```python
from build123d import *

# Parameters (mm, degrees)
ESBO_O2_R                = 2.5
ESBO_O2_R_2              = 2
RESSALTO_EXTRUS_O1_DEPTH = 3
ESBO_O3_W                = 5.4
ESBO_O3_H                = 7.4
ESBO_O3_W_2              = 3.4
ESBO_O3_H_2              = 5.4
RESSALTO_EXTRUS_O2_DEPTH = 1.2
RESSALTO_EXTRUS_O3_DEPTH = 15
CHANFRO1_SIZE            = 2
FILETE1_R                = 1.5
FILETE2_R                = 1
RESSALTO_EXTRUS_O4_DEPTH = 3
RESSALTO_EXTRUS_O5_DEPTH = 1.3
RESSALTO_EXTRUS_O6_DEPTH = 1.3
RESSALTO_EXTRUS_O7_DEPTH = 3
CHANFRO2_SIZE            = 1.5
ESBO_O10_R               = 2.5
CORTE_EXTRUS_O1_DEPTH    = 13
CHANFRO3_SIZE            = 1.5
CORTE_EXTRUS_O2_DEPTH    = 13
ESBO_O12_W               = 47.4
ESBO_O12_H               = 3
RESSALTO_EXTRUS_O8_DEPTH = 3
CHANFRO4_SIZE            = 2


# Some blends are built 0.0001 mm under size
with BuildPart() as part:
    # Esboço2 → Ressalto-extrusão1 (new body)
    with BuildSketch(Plane.XY):
        with BuildLine():
            Line((-19.293876913, 20.175), (-19.293876913, -17.425))
            Line((-19.293876913, -17.425), (-9, -17.425))
            Line((-9, -17.425), (-9, -19.425))
            Line((-9, -19.425), (38.4, -19.425))
            Line((38.4, -19.425), (38.4, -17.425))
            Line((38.4, -17.425), (42.4, -17.425))
            Line((42.4, -17.425), (42.4, 20.175))
            Line((42.4, 20.175), (62.4, 20.175))
            ThreePointArc((62.4, 20.175), (63.107106781, 19.882106781), (63.4, 19.175))
            Line((63.4, 19.175), (63.4, -20.425))
            Line((63.4, -20.425), (42.4, -20.425))
            Line((42.4, -20.425), (-19.293876913, -20.425))
            Line((-19.293876913, -20.425), (-34, -20.425))
            Line((-34, -20.425), (-34, 19.175))
            ThreePointArc((-34, 19.175), (-33.707106781, 19.882106781), (-33, 20.175))
            Line((-33, 20.175), (-19.293876913, 20.175))
        make_face()
        with Locations((-24.25, 0)):
            Circle(ESBO_O2_R, mode=Mode.SUBTRACT)
        with Locations((58.4, -14.825)):
            Circle(ESBO_O2_R_2, mode=Mode.SUBTRACT)
    extrude(amount=RESSALTO_EXTRUS_O1_DEPTH)

    # Esboço3 → Ressalto-extrusão2 (add)
    with BuildSketch(Plane(origin=(0, 0, 0), x_dir=(-1, 0, 0), z_dir=(0, 0, -1))):
        with Locations((-48.4, 11.175)):
            Rectangle(ESBO_O3_W, ESBO_O3_H)
        with Locations((-48.4, -10.825)):
            Rectangle(ESBO_O3_W, ESBO_O3_H)
        with Locations((27, 11.175)):
            Rectangle(ESBO_O3_W_2, ESBO_O3_H_2)
        with Locations((27, -10.825)):
            Rectangle(ESBO_O3_W_2, ESBO_O3_H_2)
    extrude(amount=RESSALTO_EXTRUS_O2_DEPTH)

    # Esboço4 → Ressalto-extrusão3 (add)
    with BuildSketch(Plane.XY.offset(3)):
        with BuildLine():
            Line((-34, -20.425), (63.4, -20.425))
            Line((63.4, -20.425), (63.4, -17.425))
            Line((63.4, -17.425), (61.439736831, -17.425))
            ThreePointArc((61.439736831, -17.425), (58.4, -18.825), (55.360263169, -17.425))
            Line((55.360263169, -17.425), (38.4, -17.425))
            Line((38.4, -17.425), (38.4, -19.425))
            Line((38.4, -19.425), (-9, -19.425))
            Line((-9, -19.425), (-9, -17.425))
            Line((-9, -17.425), (-34, -17.425))
            Line((-34, -17.425), (-34, -20.425))
        make_face()
    extrude(amount=RESSALTO_EXTRUS_O3_DEPTH)

    # Chanfro1
    chanfro1_edges = [part.edges().sort_by_distance(p)[0] for p in [
        (38.4, -19.425, 9),
        (-9, -19.425, 9),
    ]]
    chamfer(chanfro1_edges, length=CHANFRO1_SIZE - 0.0001)  # a hair under: the kernel refuses the full size

    # Filete1
    filete1_edges = [part.edges().sort_by_distance(p)[0] for p in [
        (61.439736831, -17.425, 10.5),
        (55.360263169, -17.425, 10.5),
    ]]
    fillet(filete1_edges, radius=FILETE1_R)

    # Filete2
    filete2_edges = [part.edges().sort_by_distance(p)[0] for p in [
        (-19.293876913, 20.175, 1.5),
        (42.4, 20.175, 1.5),
    ]]
    fillet(filete2_edges, radius=FILETE2_R)

    # Esboço6 → Ressalto-extrusão4 (add)
    with BuildSketch(Plane.ZY.offset(34)):
        Polygon((18, -17.425), (3, -2.425), (3, -17.425), align=None)
    extrude(amount=-RESSALTO_EXTRUS_O4_DEPTH)

    # Esboço7 → Ressalto-extrusão5 (add)
    with BuildSketch(Plane(origin=(63.4, 0, 0), x_dir=(0, 0, -1), z_dir=(1, 0, 0))):
        Polygon((-18, -17.425), (-3, -2.5), (-3, -17.425), align=None)
    extrude(amount=-RESSALTO_EXTRUS_O5_DEPTH)

    # Esboço8 → Ressalto-extrusão6 (add)
    with BuildSketch(Plane(origin=(-19.293876913, 0, 0), x_dir=(0, 0, -1), z_dir=(1, 0, 0))):
        Polygon((-3, -2.425), (-3, -17.425), (-18, -17.425), align=None)
    extrude(amount=-RESSALTO_EXTRUS_O6_DEPTH)

    # Esboço9 → Ressalto-extrusão7 (add)
    with BuildSketch(Plane.ZY.offset(-42.4)):
        Polygon((3, -2.425), (3, -17.425), (18, -17.425), align=None)
    extrude(amount=-RESSALTO_EXTRUS_O7_DEPTH)

    # Chanfro2
    chanfro2_edges = [part.edges().sort_by_distance(p)[0] for p in [
        (-31, -17.425, 10.5),
        (-25.796938457, -17.425, 3),
        (-20.593876913, -17.425, 10.5),
        (45.4, -17.425, 10.5),
        (-19.293876913, -17.425, 9),
        (42.4, -17.425, 9),
    ]]
    chamfer(chanfro2_edges, length=CHANFRO2_SIZE)

    # Esboço10 → Corte-extrusão1 (cut)
    with BuildSketch(Plane(origin=(0, -17.425, 0), x_dir=(1, 0, 0), z_dir=(0, 1, 0))):
        with Locations(Location((-13.396938457, -10.5, 0), (0, 0, 270))):
            Circle(ESBO_O10_R)
        with Locations(Location((50.816969722, -10.5, 0), (0, 0, 270))):
            Circle(ESBO_O10_R)
    extrude(amount=-CORTE_EXTRUS_O1_DEPTH, mode=Mode.SUBTRACT)

    # Chanfro3
    # the kernel refuses this chamfer: 1.5 mm, written as the material it takes off along each edge
    with BuildSketch(Plane(origin=(-13.396938457, -17.425, 10.5), x_dir=(0, 0, 1), z_dir=(-1, 0, 0))) as chanfro3_piece_1:
        Polygon((2.5 + CHANFRO3_SIZE, 0), (2.5, -CHANFRO3_SIZE), (2.5, 0), align=None)
    revolve(axis=Axis((-13.396938457, -17.425, 10.5), (0, 1, 0)), mode=Mode.SUBTRACT)
    with BuildSketch(Plane(origin=(50.816969722, -17.425, 10.5), x_dir=(0, 0, 1), z_dir=(-1, 0, 0))) as chanfro3_piece_2_section:
        Polygon((2.5 + CHANFRO3_SIZE, 0), (2.5, -CHANFRO3_SIZE), (2.5, 0), align=None)
    chanfro3_piece_2 = revolve(axis=Axis((50.816969722, -17.425, 10.5), (0, 1, 0)), mode=Mode.PRIVATE)
    chanfro3_piece_2 = split(chanfro3_piece_2, bisect_by=Plane(origin=(50.475171982, -21.000171982, 8.459359331), z_dir=(0.7071067811865476, 0.7071067811865476, 0)), keep=Keep.TOP, mode=Mode.PRIVATE)
    add(chanfro3_piece_2, mode=Mode.SUBTRACT)

    # Esboço11 → Corte-extrusão2 (cut)
    with BuildSketch(Plane(origin=(0, -19.425, 0), x_dir=(1, 0, 0), z_dir=(0, 1, 0))):
        with BuildLine():
            Line((1, -2.5), (28.4, -2.5))
            ThreePointArc((28.4, -2.5), (32.4, -6.5), (28.4, -10.5))
            Line((28.4, -10.5), (1, -10.5))
            ThreePointArc((1, -10.5), (-3, -6.5), (1, -2.5))
        make_face()
    extrude(amount=-CORTE_EXTRUS_O2_DEPTH, mode=Mode.SUBTRACT)

    # Esboço12 → Ressalto-extrusão8 (add)
    with BuildSketch(Plane.XY.offset(18)):
        with Locations((14.7, -18.925)):
            Rectangle(ESBO_O12_W, ESBO_O12_H)
    extrude(amount=-RESSALTO_EXTRUS_O8_DEPTH)

    # Chanfro4
    chanfro4_edges = [part.edges().sort_by_distance(p)[0] for p in [
        (14.7, -19.425, 15),
    ]]
    chamfer(chanfro4_edges, length=CHANFRO4_SIZE - 0.0001)  # a hair under: the kernel refuses the full size


solid = part.part
```
The listing builds one solid part. Answer for the finished solid, in the listing's coordinates (mm). A direction names the side the tool comes from. Round coordinates to 2 decimals unless told otherwise and drop trailing zeros. Loops run counter-clockwise (first coordinate to the right, second up) from the corner with the lowest first, then second, coordinate; pieces in that order, holes last. Notation, with made-up numbers: (18, -14) - (59, -14) arc R30 cw to (59, 13) - close; hole circle Ø3 at (-30, 46.5). An arc over 180 degrees is marked (long way). Use one line per item in the form item = value. Start each with the question number.
1. The part is cut by section D-D on x = -24.25. Determine the outline of the cut face in (y, z) (3 decimals), then the cut area to 3 significant figures.
2. A tool of negligible diameter and unlimited length cuts with its end or side. For faces 3 (the face through (46.254, -16.779, 10.395)), 4 (the face through (7, -17.425, 16)), 5 (the face through (45.4, -12, 7)), from which of +Z, -Z, +X, -X, +Y, -Y can it reach the whole face along a straight path? Write none if from no direction.
3. Given pin 1 Ø1.3 at (x, z) = (49.5, -1) entering from -Y (3 decimals); pin 2 Ø9 at (x, z) = (9, 7.5) entering from +Y (3 decimals); pin 3 Ø5 at (x, y) = (41.5, -8.5) entering from -Z; pin 4 Ø5 at (y, z) = (16, 5) entering from +X, each flat-ended and moving along its own axis, determine where each tip first touches the part or whether it passes through.
4. The part is cut by section A-A on y = 0. Determine the outline of the cut face in (x, z), then the cut area to 3 significant figures.
5. For a pull along X with two mould halves and no side action, classify faces 1 (the face through (14, -19, 18)), 2 (the face through (37.386, -18.439, 7.395)) as pulls with the +X half, pulls with the -X half, needs draft (parallel to the pull), parting line crosses it, or undercut.
6. The part is cut by section C-C on y = -9. Determine the outline of the cut face in (x, z) (3 decimals).
7. Consider line 1 (X direction, y = -15, z = 11); line 2 (X direction, y = -16, z = 5.5) (3 decimals); line 3 (Y direction, x = 58.4, z = 1.25) (3 decimals). Determine where each line is inside the solid, lowest interval first. Write a range as [from, to].
Geometry check:
q1.outline = (-20.425, 0) - (-2.5, 0) - (-2.5, 3) - (-15.925, 3) - (-17.425, 4.5) - (-17.425, 18) - (-20.425, 18) - close; (2.5, 0) - (20.175, 0) - (20.175, 3) - (2.5, 3) - close
q1.area = 153 mm^2
q2.face_3 = +Y
q2.face_4 = +Z, -Z, +Y
q2.face_5 = +Z, +Y
q3.pin_1 = -14.525
q3.pin_2 = -19.425
q3.pin_3 = 0
q3.pin_4 = 63.4
q4.outline = (-34, 0) - (-26.75, 0) - (-26.75, 3) - (-34, 3) - close; (-21.75, 0) - (-19.29, 0) - (-19.29, 3) - (-21.75, 3) - close; (42.4, 0) - (63.4, 0) - (63.4, 3) - (42.4, 3) - close
q4.area = 92.1 mm^2
q5.face_1 = needs draft
q5.face_2 = undercut
q6.outline = (-34, 0) - (-28.7, 0) - (-28.7, -1.2) - (-25.3, -1.2) - (-25.3, 0) - (-19.294, 0) - (-19.294, 9.575) - (-20.594, 9.575) - (-20.594, 3) - (-31, 3) - (-31, 9.575) - (-34, 9.575) - close; (42.4, 0) - (45.7, 0) - (45.7, -1.2) - (51.1, -1.2) - (51.1, 0) - (63.4, 0) - (63.4, 9.533) - (62.1, 9.533) - (62.1, 3) - (45.4, 3) - (45.4, 9.575) - (42.4, 9.575) - close
q7.line_1 = [-34, -31], [-20.59, -19.29], [42.4, 45.4], [62.1, 63.4]
q7.line_2 = [-34, -30.925], [-20.669, -19.219], [42.325, 45.475], [62.1, 63.4]
q7.line_3 = [-20.425, -16.825], [-12.825, 20.175]
